from build123d import *

# Parameters (mm, degrees)
F2_DEPTH = 7.62
F3_R     = 25.4
F4_DEPTH = 3.81
F5_SIZE  = 3.7338
F6_R     = 1.27
F9_D     = 5.588
F9_DEPTH = 127
F9_TIP   = 1.6788045696


with BuildPart() as f2:
    # F1 (on Top) → F2 (new body)
    with BuildSketch(Plane.XY):
        Polygon((-3.0674997251, -7.4159256183), (0, -32.8098908067), (3.0712168664, -7.4155884795), (14.2346806824, -14.2299178988), (7.4049378745, -3.0691174325), (20.1237425208, 0), (7.4238278903, 3.0710902065), (14.2239863053, 14.2202461138), (3.068682272, 7.4126794934), (0, 32.8086838126), (-3.0691300053, 7.4164932594), (-14.2189133912, 14.2328040674), (-7.413723506, 3.0703686643), (-20.1198514551, 0), (-7.4060442857, -3.0691174325), (-14.2189133912, -14.1971036792), align=None)
    extrude(amount=F2_DEPTH)

    # F3 (on Top) → F4 (join)
    with BuildSketch(Plane.XY):
        Circle(F3_R)
    extrude(amount=F4_DEPTH)

    # F5
    f5_edges = [f2.edges().sort_by_distance(p)[0] for p in [
        (-10.812479, -8.633111, 7.62),
        (-8.643207, -10.806515, 7.62),
        (-1.53375, -20.112908, 7.62),
        (1.535608, -20.11274, 7.62),
        (8.652949, -10.822753, 7.62),
        (10.819809, -8.649518, 7.62),
        (13.76434, -1.534559, 7.62),
        (13.773785, 1.535545, 7.62),
        (10.823907, 8.645668, 7.62),
        (8.646334, 10.816463, 7.62),
        (1.534341, 20.110682, 7.62),
        (-1.534565, 20.112589, 7.62),
        (-8.644022, 10.824649, 7.62),
        (-10.816318, 8.651586, 7.62),
        (-13.766787, 1.535184, 7.62),
        (-13.762948, -1.534559, 7.62),
    ]]
    chamfer(f5_edges, length=F5_SIZE)

    # F6
    f6_edges = [f2.edges().sort_by_distance(p)[0] for p in [
        (25.4, 0.000476, 3.81),
        (-25.4, -0.000198, 3.81),
    ]]
    fillet(f6_edges, radius=F6_R)

    # F9 (one way)
    with BuildSketch(Plane.XY.offset(3.81)):
        with Locations((-20.8135005087, 0), (20.8601150662, 0)):
            Circle(F9_D / 2)
    extrude(amount=-F9_DEPTH, mode=Mode.SUBTRACT)
    with Locations(Plane.XY.offset(3.81)):
        with Locations((-20.8135005087, 0), (20.8601150662, 0)):
            with Locations((0, 0, -(F9_DEPTH + F9_TIP / 2))):  # 118° drill point
                Cone(0, F9_D / 2, F9_TIP, mode=Mode.SUBTRACT)


solid = f2.part
Read the model definition and answer for the solid it produces. Units are mm, in the model's axes. A direction names the side the tool comes from. Coordinates: 2 decimals unless noted, no trailing zeros. Order: outer loops, then holes, each group sorted by start corner. A loop starts at its lowest first (then second) coordinate and runs counter-clockwise, first axis right, second up. Notation, with made-up numbers: M 19.25,54.5 L 45.25,54.5 A26 cw 45.25,91.5 Z; hole C 5.5,77.5 d4. An arc over 180 degrees is marked long. Put each result on its own line as item: value. Start each with the question number.
Item 1: Given pin 1 Ø0.8 at (x, y) = (18.5, 0) entering from -Z; pin 2 Ø5 at (x, y) = (-17, 11) entering from +Z; pin 3 Ø2 at (x, z) = (16.5, 1.5) entering from +Y, each flat-ended and moving along its own axis, determine where each tip first touches the part or whether it passes through.
Item 2: The mould has two halves that part along Y. Classify faces 6 (the face through (-13, -5, 3.81)), 7 (the face through (0, 0, 0)), 8 (the face through (-0.91, -13.39, 5.31)): +Y half, -Y half, draft (parallel to the pull), parting line (faces both ways), or undercut.
Item 3: Consider probe 1 along X at (y, z) = (0, 1.75); probe 2 along Y at (x, z) = (-8, 2.25); probe 3 along Z at (x, y) = (3, 18). Determine where each line is inside the solid, lowest interval first. Write a range as [from, to].
Item 4: For faces 1 (the face through (7.111, 5.397, 5.364)), 2 (the face through (-9.09, -1.2, 5.31)), 3 (the face through (-25.394, 0.546, 1.252)), 4 (the face through (0.86, -13.82, 5.31)), 5 (the face through (25.394, -0.545, 1.252)), determine the directions among +Z, -Z, +X, -X, +Y, -Y from which every point of the face is accessible in a straight line to the end or side of a thin tool.
Item 5: Section A-A, the plane z = 6.5 is taken. Determine the outline of the cut face in (x, y), plus the area to 3 significant figures.
Computed:
1. pin 1: stops at z = 3.81
1. pin 2: stops at z = 3.81
1. pin 3: stops at y = 20.12
2. face 6: undercut
2. face 7: draft
2. face 8: -Y half
3. probe 1: x = [-25.4, -23.61], [-18.02, 18.07], [23.65, 25.4]
3. probe 2: y = [-24.11, 24.11]
3. probe 3: z = [0, 3.81]
4. face 1: +Z, +X
4. face 2: +Z, -X
4. face 3: +Z, -Z, -X
4. face 4: +Z, -Y
4. face 5: +Z, -Z, +X
5. outline: M -8.99,0 L -3.3,-1.37 L -6.35,-6.35 L -0.96,-3.07 L 0,-11.03 L 0.96,-3.07 L 6.35,-6.36 L 3.3,-1.37 L 8.99,0 L 3.33,1.37 L 6.37,6.37 L 0.96,3.06 L 0,11.02 L -0.96,3.06 L -6.36,6.37 L -3.32,1.37 Z
5. area: 97.3 mm2
